```python
from build123d import *

# Parameters (mm, degrees)
SKETCH1_W           = 262.6868
SKETCH1_H           = 130.175
BOSS_EXTRUDE1_DEPTH = 4.3434
SKETCH2_W           = 19.05
SKETCH2_H           = 8.6868
CUT_EXTRUDE1_DEPTH  = 147.650388692
SKETCH3_W           = 8.6868
SKETCH3_H           = 19.05
CUT_EXTRUDE3_DEPTH  = 147.650388692


with BuildPart() as part:
    # Sketch1 → Boss-Extrude1 (new body)
    with BuildSketch(Plane.XY):
        Rectangle(SKETCH1_W, SKETCH1_H)
    extrude(amount=BOSS_EXTRUDE1_DEPTH)

    # Sketch2 → Cut-Extrude1 (cut, through all)
    with BuildSketch(Plane.XY.offset(4.3434)):
        with Locations((-50.8, 65.0875)):
            Rectangle(SKETCH2_W, SKETCH2_H)
        with Locations((0, 65.0875)):
            Rectangle(SKETCH2_W, SKETCH2_H)
        with Locations((50.8, 65.0875)):
            Rectangle(SKETCH2_W, SKETCH2_H)
        with Locations((101.6, 65.0875)):
            Rectangle(SKETCH2_W, SKETCH2_H)
        with Locations((-101.6, 65.0875)):
            Rectangle(SKETCH2_W, SKETCH2_H)
    extrude(amount=-CUT_EXTRUDE1_DEPTH, mode=Mode.SUBTRACT)

    # Sketch3 → Cut-Extrude3 (cut, through all)
    with BuildSketch(Plane.XY.offset(4.3434)):
        with Locations((-131.3434, -25.4)):
            Rectangle(SKETCH3_W, SKETCH3_H)
        with Locations((-131.3434, 25.4)):
            Rectangle(SKETCH3_W, SKETCH3_H)
    cut_extrude3 = extrude(amount=-CUT_EXTRUDE3_DEPTH, mode=Mode.SUBTRACT)

    # Mirror1: Cut-Extrude3 across plane
    add(cut_extrude3.mirror(Plane(origin=(0, 0, 0), x_dir=(0, 0, 1), z_dir=(1, 0, 0))), mode=Mode.SUBTRACT)


solid = part.part
```
Could you check a few things on this model? Use its own coordinates, in mm. Coordinates: 2 decimals unless noted, no trailing zeros. Write each loop counter-clockwise with the first axis right and the second up, starting at its lowest first coordinate (ties: lowest second). Pieces come first, ordered by that corner, then holes. Notation, with made-up numbers: (27, 3) -> (72, 3) arc R25 ccw to (72, 17) -> close; hole circle Ø9 at (9, -34.75). An arc over 180 degrees is marked (long way). One line per question, with ' | ' between items. Start each with the question number.
1. If we section it at A-A (x = -101): Please give me the cut outline in (y, z).
2. If we section it at B-B (y = -30.5): Please give me the cut outline in (x, z).
3. Will this pin go through, and if not, where does the flat tip stop? P1, Ø1.3, axis at x = -104, z = 3, coming from the +Y side.
4. Please list where these lines run through material, in increasing order: line 1 along Y through (x, z) = (-42, 1.95); line 2 along X through (y, z) = (-28, 1.3).
Return value:
1) outline: (-65.09, 0) -> (60.74, 0) -> (60.74, 4.34) -> (-65.09, 4.34) -> close
2) outline: (-127, 0) -> (127, 0) -> (127, 4.34) -> (-127, 4.34) -> close
3) P1: stops at y = 60.74
4) line 1: y = -65.09 to 60.74 | line 2: x = -127 to 127
